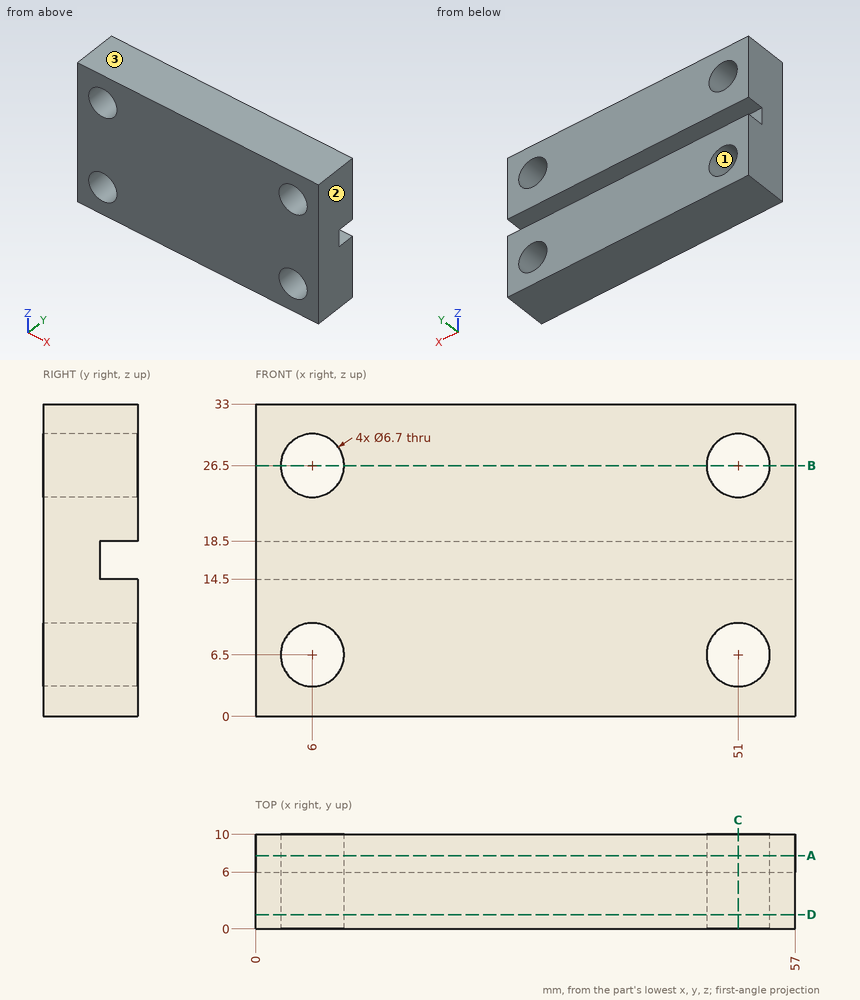
Geometry check sheet. Reference: drawing and pictorial views, mm from the part's lowest x, y, z. Round coordinates to 2 decimals unless told otherwise and drop trailing zeros. Loops run counter-clockwise (first coordinate to the right, second up) from the corner with the lowest first, then second, coordinate; pieces in that order, holes last. Notation, with made-up numbers: (89.5, -28) - (139.5, -28) arc R16 ccw to (139.5, -14) - close; hole circle Ø2 at (87.25, 44). An arc over 180 degrees is marked (long way). Use a Markdown table: item, result. Add a question column.
1. Section check B-B, the plane z = 26.5. Record the boundary of the cut face in (x, y).
2. Thickness scan on probe 1 along Z at (x, y) = (51, 7.5); probe 2 along Z at (x, y) = (51, 5.5); probe 3 along Z at (x, y) = (50, 3.5). Record the ranges inside material, lowest first. Write a range as [from, to].
3. Release check for a two-part mould opening along Z. For the marked faces 1, 2 and 3 record: released by +Z, released by -Z, zero draft, split by the parting line, or undercut.
4. Section check A-A, the plane y = 7.75. Record the boundary of the cut face in (x, z), plus the area to 3 significant figures.
5. Section check C-C, the plane x = 51. Record the boundary of the cut face in (y, z), plus the area to 3 significant figures.
6. Section check D-D, the plane y = 1.5. Record the boundary of the cut face in (x, z).
Checks:
| question | item | result |
|---|---|---|
| 1 | outline | (0, 0) - (2.65, 0) - (2.65, 10) - (0, 10) - close; (9.35, 0) - (47.65, 0) - (47.65, 10) - (9.35, 10) - close; (54.35, 0) - (57, 0) - (57, 10) - (54.35, 10) - close |
| 2 | probe 1 | z = [0, 3.15], [9.85, 14.5], [18.5, 23.15], [29.85, 33] |
| 2 | probe 2 | z = [0, 3.15], [9.85, 23.15], [29.85, 33] |
| 2 | probe 3 | z = [0, 3.3], [9.7, 23.3], [29.7, 33] |
| 3 | face 1 | undercut |
| 3 | face 2 | zero draft |
| 3 | face 3 | released by +Z |
| 4 | outline | (0, 0) - (57, 0) - (57, 14.5) - (0, 14.5) - close; (0, 18.5) - (57, 18.5) - (57, 33) - (0, 33) - close; hole circle Ø6.7 at (6, 6.5); hole circle Ø6.7 at (6, 26.5); hole circle Ø6.7 at (51, 6.5); hole circle Ø6.7 at (51, 26.5) |
| 4 | area | 1,510 mm^2 |
| 5 | outline | (0, 0) - (10, 0) - (10, 3.15) - (0, 3.15) - close; (0, 9.85) - (10, 9.85) - (10, 14.5) - (6, 14.5) - (6, 18.5) - (10, 18.5) - (10, 23.15) - (0, 23.15) - close; (0, 29.85) - (10, 29.85) - (10, 33) - (0, 33) - close |
| 5 | area | 180 mm^2 |
| 6 | outline | (0, 0) - (57, 0) - (57, 33) - (0, 33) - close; hole circle Ø6.7 at (6, 6.5); hole circle Ø6.7 at (6, 26.5); hole circle Ø6.7 at (51, 6.5); hole circle Ø6.7 at (51, 26.5) |
